Geometry: final body of the model. Coordinates: model frame, mm. A direction names the side the tool comes from. Coordinates: 2 decimals unless noted, no trailing zeros. Write each loop counter-clockwise with the first axis right and the second up, starting at its lowest first coordinate (ties: lowest second). Pieces come first, ordered by that corner, then holes. Notation, with made-up numbers: (-19, 2) -> (37, 2) arc R32 ccw to (37, 29) -> close; hole circle Ø8 at (31, -15). An arc over 180 degrees is marked (long way). Answer as a JSON object with one key per item and string values. Group by question number.
```python
from build123d import *

# Parameters (mm, degrees)
SKETCH_1_R      = 3.5
SKETCH_1_R_2    = 2.5
EXTRUDE_1_DEPTH = 4.8
SKETCH_2_R      = 1.5
SKETCH_2_R_2    = 1
EXTRUDE_2_DEPTH = 2.5


with BuildPart() as part:
    # 草图1 → 凸台-拉伸1 (new body)
    with BuildSketch(Plane(origin=(0, 0, 0), x_dir=(1, 0, 0), z_dir=(0, 1, 0))):
        with Locations(Location((0, 0, 0), (0, 0, 270))):
            Circle(SKETCH_1_R)
        with Locations(Location((0, 0, 0), (0, 0, 270))):
            Circle(SKETCH_1_R_2, mode=Mode.SUBTRACT)
    extrude(amount=EXTRUDE_1_DEPTH)

    # 草图2 → 凸台-拉伸2 (add)
    with BuildSketch(Plane.XZ):
        with BuildLine():
            Line((-13.702785185, 2.311120544), (-0.305925926, 3.486604269))
            ThreePointArc((-0.305925926, 3.486604269), (3.5, 0), (-0.305925926, -3.486604269))
            Line((-0.305925926, -3.486604269), (-13.702785185, -2.311120544))
            ThreePointArc((-13.702785185, -2.311120544), (-15.82, 0), (-13.702785185, 2.311120544))
        make_face()
        with Locations(Location((0, 0, 0), (0, 0, 270))):
            Circle(SKETCH_2_R, mode=Mode.SUBTRACT)
        with Locations(Location((-13.5, 0, 0), (0, 0, 270))):
            Circle(SKETCH_2_R_2, mode=Mode.SUBTRACT)
        with Locations(Location((-11, 0, 0), (0, 0, 270))):
            Circle(SKETCH_2_R_2, mode=Mode.SUBTRACT)
        with Locations(Location((-8.5, 0, 0), (0, 0, 270))):
            Circle(SKETCH_2_R_2, mode=Mode.SUBTRACT)
        with Locations(Location((-6, 0, 0), (0, 0, 270))):
            Circle(SKETCH_2_R_2, mode=Mode.SUBTRACT)
    extrude(amount=-EXTRUDE_2_DEPTH)


solid = part.part
```
Item 1: Section C-C on y = 0.7. Output: boundary loops of the cut face in (x, z).
Item 2: Section B-B on z = 0. Give the number of separate pieces and of enclosed holes in the cut face, then the cut area to 3 significant figures.
Item 3: Set-up query: faces 4 (the flat face through (-7.1, 1.23, 2.89)), 5 (the cylindrical face through (-2.44, 3.63, -0.54)). Return all of +Z, -Z, +X, -X, +Y, -Y with unobstructed straight access to the full face (end or side cutting, diameter ignored); none if empty.
Item 4: Mould query, pull axis X, two halves, no side actions, for faces 1 (the cylindrical face through (-5, 1, 0)), 2 (the flat face through (-2, 4.8, 2)), 3 (the flat face through (-6.911, 1.232, -2.907)). Classes: +X half, -X half, draft (parallel to the pull), parting line (faces both ways), or undercut.
Item 5: Contact query for flat-ended pins moving along their axis: pin 1 (4 mm diameter, centred on x = -10.5, z = -2.5, fed in from +Y); pin 2 (1.2 mm diameter, centred on x = -6, z = 0, fed in from -Y); pin 3 (1.5 mm diameter, centred on x = -1, y = 2.5, fed in from -Z); pin 4 (1.5 mm diameter, centred on x = -1, y = 0.5, fed in from +Z). Output: stop coordinate, or through.
Item 6: Section D-D on z = -1.25. Output: boundary loops of the cut face in (x, y).
Item 7: Section A-A on x = 0. Output: boundary loops of the cut face in (y, z), then the cut area to 3 significant figures.
Item 8: Ray query, L1, parallel to X at y = 1.45, z = 0; L2, parallel to Z at x = 0, y = 3.7; L3, parallel to Y at x = -9, z = -1. Return the intervals inside material, ascending. Write a range as [from, to].
Answer sheet:
{
 "1": {"outline": "(-13.7, -2.31) -> (-0.31, -3.49) arc R3.5 ccw (long way) to (-0.31, 3.49) -> (-13.7, 2.31) arc R2.32 ccw to start; hole circle Ø2 at (-13.5, 0); hole circle Ø2 at (-11, 0); hole circle Ø2 at (-8.5, 0); hole circle Ø2 at (-6, 0); hole circle Ø3 at (0, 0)"},
 "2": {"separate pieces": "6", "enclosed holes": "0", "area": "25.4 mm^2"},
 "3": {"face 4": "+Z, -X, +Y, -Y", "face 5": "+Y"},
 "4": {"face 1": "undercut", "face 2": "draft", "face 3": "-X half"},
 "5": {"pin 1": "stops at y = 2.5", "pin 2": "passes through", "pin 3": "stops at z = -3.49", "pin 4": "stops at z = 3.49"},
 "6": {"outline": "(-15.45, 0) -> (-0.83, 0) -> (-0.83, 2.5) -> (-2.17, 2.5) -> (-2.17, 4.8) -> (-3.27, 4.8) -> (-3.27, 2.5) -> (-15.45, 2.5) -> close; (0.83, 0) -> (3.27, 0) -> (3.27, 4.8) -> (2.17, 4.8) -> (2.17, 2.5) -> (0.83, 2.5) -> close"},
 "7": {"outline": "(0, -3.5) -> (4.8, -3.5) -> (4.8, -2.5) -> (2.5, -2.5) -> (2.5, -1.5) -> (0, -1.5) -> close; (0, 1.5) -> (2.5, 1.5) -> (2.5, 2.5) -> (4.8, 2.5) -> (4.8, 3.5) -> (0, 3.5) -> close", "area": "14.6 mm^2"},
 "8": {"L1": "x = [-15.82, -14.5], [-12.5, -12], [-10, -9.5], [-7.5, -7], [-5, -1.5], [1.5, 3.5]", "L2": "z = [-3.5, -2.5], [2.5, 3.5]", "L3": "y = [0, 2.5]"}
}
